from build123d import *

# Parameters (mm, degrees)
CHAMFER1_SIZE                   = 2
BOSS_EXTRUDE1_DEPTH             = 70
CHAMFER2_SIZE                   = 14
SKETCH3_R                       = 5
CUT_EXTRUDE1_DEPTH              = 70
CIRPATTERN1_COUNT               = 4
CHAMFER2_OF_CIRPATTERN1_SIZE    = 14
CUT_EXTRUDE2_START              = 70
CUT_EXTRUDE2_DEPTH              = 70
CUT_EXTRUDE3_DEPTH              = 70
CIRPATTERN2_COUNT               = 2
CIRPATTERN2_ANGLE               = 10
CIRPATTERN2_THE_OTHER_WAY_COUNT = 2
CIRPATTERN2_THE_OTHER_WAY_ANGLE = 10
CIRPATTERN3_COUNT               = 4
CIRPATTERN3_COPY_1_DEPTH        = 70
CIRPATTERN3_COPY_2_DEPTH        = 70
CIRPATTERN3_COPY_3_DEPTH        = 70
CIRPATTERN3_COPY_4_DEPTH        = 70
CIRPATTERN3_COPY_5_DEPTH        = 70
CIRPATTERN3_COPY_6_DEPTH        = 70
CUT_SWEEP2_PROFILE_R            = 0.5
CUT_SWEEP3_PROFILE_R            = 0.5
CUT_EXTRUDE4_START              = -10
SKETCH27_R                      = 37.5
CUT_EXTRUDE4_DEPTH              = 10


with BuildPart() as part:
    # Sketch1 → Revolve1 (revolve)
    with BuildSketch(Plane.XY, mode=Mode.PRIVATE) as revolve1_sk:
        Polygon((0, 0), (-50, 0), (-50, 28), (-37.5, 28), (-37.5, 31), (-5, 31), (-5, 41), (0, 41), align=None)
    revolve(revolve1_sk.sketch.rotate(Axis((0, 0, 0), (0, 1, 0)), 270), axis=Axis((0, 0, 0), (0, 1, 0)))

    # Chamfer1
    chamfer1_edges = [part.edges().sort_by_distance(p)[0] for p in [
        (0, 31, 37.5),
        (0, 28, 50),
    ]]
    chamfer(chamfer1_edges, length=CHAMFER1_SIZE)

    # Sketch2 → Boss-Extrude1 (add)
    with BuildSketch(Plane.XY):
        Polygon((12.5, 0), (-12.5, 0), (-12.5, 26), (-10.5, 26), (-10.5, 2), (10.5, 2), (10.5, 26), (12.5, 26), align=None)
    boss_extrude1 = extrude(amount=BOSS_EXTRUDE1_DEPTH)

    # Chamfer2
    chamfer2_edges = [part.edges().sort_by_distance(p)[0] for p in [
        (-11.5, 26, 70),
        (11.5, 26, 70),
    ]]
    chamfer(chamfer2_edges, length=CHAMFER2_SIZE)

    # Sketch3 → Cut-Extrude1 (cut)
    with BuildSketch(Plane(origin=(0, 31, 0), x_dir=(1, 0, 0), z_dir=(0, 1, 0))):
        with Locations(Location((0, -60, 0), (0, 0, 270))):
            Circle(SKETCH3_R)
    cut_extrude1 = extrude(amount=-CUT_EXTRUDE1_DEPTH, mode=Mode.SUBTRACT)

    # CirPattern1: Boss-Extrude1, Cut-Extrude1 ×4 about axis
    cirpattern1_axis = Axis((0, 0, 0), (0, 1, 0))
    add([boss_extrude1.rotate(cirpattern1_axis, i * 360 / CIRPATTERN1_COUNT) for i in range(1, CIRPATTERN1_COUNT)])
    add([cut_extrude1.rotate(cirpattern1_axis, i * 360 / CIRPATTERN1_COUNT) for i in range(1, CIRPATTERN1_COUNT)], mode=Mode.SUBTRACT)

    # Chamfer2 of CirPattern1
    chamfer2_of_cirpattern1_edges = [part.edges().sort_by_distance(p)[0] for p in [
        (70, 26, 11.5),
        (70, 26, -11.5),
        (11.5, 26, -70),
        (-11.5, 26, -70),
        (-70, 26, -11.5),
        (-70, 26, 11.5),
    ]]
    chamfer(chamfer2_of_cirpattern1_edges, length=CHAMFER2_OF_CIRPATTERN1_SIZE)

    # Sketch4 → Cut-Extrude2 (cut)
    with BuildSketch(Plane(origin=(0, 0, 0), x_dir=(1, 0, 0), z_dir=(0, 1, 0)).offset(CUT_EXTRUDE2_START)):
        with BuildLine():
            Line((23.02513458, -42.117017672), (23.12024219, -44.333445626))
            ThreePointArc((23.12024219, -44.333445626), (35.355339059, -35.355339059), (44.333445626, -23.12024219))
            Line((44.333445626, -23.12024219), (42.117017672, -23.02513458))
            ThreePointArc((42.117017672, -23.02513458), (33.941125497, -33.941125497), (23.02513458, -42.117017672))
        make_face()
    cut_extrude2 = extrude(amount=-CUT_EXTRUDE2_DEPTH, mode=Mode.SUBTRACT)

    # Sketch5 → Cut-Extrude3 (cut)
    with BuildSketch(Plane(origin=(0, 0, 0), x_dir=(1, 0, 0), z_dir=(0, 1, 0))):
        Polygon((30.939685977, -33.941125497), (34.034072747, -36.941125497), (36.942565017, -33.941125497), (33.848178247, -30.941125497), align=None)
    cut_extrude3 = extrude(amount=CUT_EXTRUDE3_DEPTH, mode=Mode.SUBTRACT)

    # CirPattern2: Cut-Extrude3 ×2 about axis
    cirpattern2_axis = Axis((0, 0, 0), (0, 1, 0))
    for i in range(1, CIRPATTERN2_COUNT):
        add(cut_extrude3.rotate(cirpattern2_axis, i * CIRPATTERN2_ANGLE / (CIRPATTERN2_COUNT - 1)), mode=Mode.SUBTRACT)

    # CirPattern2 the other way: Cut-Extrude3 ×2 about axis
    cirpattern2_the_other_way_axis = Axis((0, 0, 0), (0, -1, 0))
    for i in range(1, CIRPATTERN2_THE_OTHER_WAY_COUNT):
        add(cut_extrude3.rotate(cirpattern2_the_other_way_axis, i * CIRPATTERN2_THE_OTHER_WAY_ANGLE / (CIRPATTERN2_THE_OTHER_WAY_COUNT - 1)), mode=Mode.SUBTRACT)

    # CirPattern3: Cut-Extrude2, Cut-Extrude3 ×4 about axis
    cirpattern3_axis = Axis((0, 0, 0), (0, 1, 0))
    add([cut_extrude2.rotate(cirpattern3_axis, i * 360 / CIRPATTERN3_COUNT) for i in range(1, CIRPATTERN3_COUNT)], mode=Mode.SUBTRACT)
    add([cut_extrude3.rotate(cirpattern3_axis, i * 360 / CIRPATTERN3_COUNT) for i in range(1, CIRPATTERN3_COUNT)], mode=Mode.SUBTRACT)

    # CirPattern3 copy 1 sketch → CirPattern3 copy 1 (cut)
    with BuildSketch(Plane(origin=(0, 0, 0), x_dir=(-0.1736481776669307, 0, -0.984807753012208), z_dir=(0, 1, 0))):
        Polygon((30.939685977, -33.941125497), (34.034072747, -36.941125497), (36.942565017, -33.941125497), (33.848178247, -30.941125497), align=None)
    extrude(amount=CIRPATTERN3_COPY_1_DEPTH, mode=Mode.SUBTRACT)

    # CirPattern3 copy 2 sketch → CirPattern3 copy 2 (cut)
    with BuildSketch(Plane(origin=(0, 0, 0), x_dir=(-0.984807753012208, 0, 0.17364817766693064), z_dir=(0, 1, 0))):
        Polygon((30.939685977, -33.941125497), (34.034072747, -36.941125497), (36.942565017, -33.941125497), (33.848178247, -30.941125497), align=None)
    extrude(amount=CIRPATTERN3_COPY_2_DEPTH, mode=Mode.SUBTRACT)

    # CirPattern3 copy 3 sketch → CirPattern3 copy 3 (cut)
    with BuildSketch(Plane(origin=(0, 0, 0), x_dir=(0.17364817766693055, 0, 0.984807753012208), z_dir=(0, 1, 0))):
        Polygon((30.939685977, -33.941125497), (34.034072747, -36.941125497), (36.942565017, -33.941125497), (33.848178247, -30.941125497), align=None)
    extrude(amount=CIRPATTERN3_COPY_3_DEPTH, mode=Mode.SUBTRACT)

    # CirPattern3 copy 4 sketch → CirPattern3 copy 4 (cut)
    with BuildSketch(Plane(origin=(0, 0, 0), x_dir=(0.1736481776669308, 0, -0.984807753012208), z_dir=(0, 1, 0))):
        Polygon((30.939685977, -33.941125497), (34.034072747, -36.941125497), (36.942565017, -33.941125497), (33.848178247, -30.941125497), align=None)
    extrude(amount=CIRPATTERN3_COPY_4_DEPTH, mode=Mode.SUBTRACT)

    # CirPattern3 copy 5 sketch → CirPattern3 copy 5 (cut)
    with BuildSketch(Plane(origin=(0, 0, 0), x_dir=(-0.984807753012208, 0, -0.17364817766693086), z_dir=(0, 1, 0))):
        Polygon((30.939685977, -33.941125497), (34.034072747, -36.941125497), (36.942565017, -33.941125497), (33.848178247, -30.941125497), align=None)
    extrude(amount=CIRPATTERN3_COPY_5_DEPTH, mode=Mode.SUBTRACT)

    # CirPattern3 copy 6 sketch → CirPattern3 copy 6 (cut)
    with BuildSketch(Plane(origin=(0, 0, 0), x_dir=(-0.17364817766693094, 0, 0.984807753012208), z_dir=(0, 1, 0))):
        Polygon((30.939685977, -33.941125497), (34.034072747, -36.941125497), (36.942565017, -33.941125497), (33.848178247, -30.941125497), align=None)
    extrude(amount=CIRPATTERN3_COPY_6_DEPTH, mode=Mode.SUBTRACT)

    # Cut-Sweep2: sweep along a path in Sketch15
    with BuildLine(Plane(origin=(0, 28, 0), x_dir=(1, 0, 0), z_dir=(0, 1, 0))) as cut_sweep2_path:
        CenterArc((0, 0), 44, 0, 360)
    # Cut-Sweep2 profile (on start of the path) → Cut-Sweep2 (sweep, cut)
    with BuildSketch(Plane(origin=(44, 28, 0), x_dir=(-1, 0, 0), z_dir=(0, 0, -1))):
        Circle(CUT_SWEEP2_PROFILE_R)
    sweep(path=cut_sweep2_path.line, mode=Mode.SUBTRACT)

    # Cut-Sweep3: sweep along a path in Sketch14
    with BuildLine(Plane(origin=(0, 28, 0), x_dir=(1, 0, 0), z_dir=(0, 1, 0))) as cut_sweep3_path:
        CenterArc((0, 0), 41, 0, 360)
    # Cut-Sweep3 profile (on start of the path) → Cut-Sweep3 (sweep, cut)
    with BuildSketch(Plane(origin=(41, 28, 0), x_dir=(-1, 0, 0), z_dir=(0, 0, -1))):
        Circle(CUT_SWEEP3_PROFILE_R)
    sweep(path=cut_sweep3_path.line, mode=Mode.SUBTRACT)

    # Sketch27 → Cut-Extrude4 (cut)
    with BuildSketch(Plane.XZ.offset(CUT_EXTRUDE4_START)):
        with Locations(Location((0, 0, 0), (0, 0, 270))):
            Circle(SKETCH27_R)
    extrude(amount=CUT_EXTRUDE4_DEPTH, mode=Mode.SUBTRACT)


solid = part.part
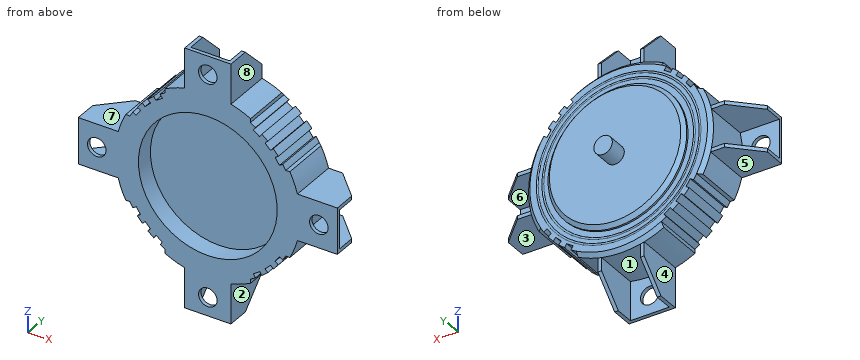
The listing builds one solid part. Answer for the finished solid, in the listing's coordinates (mm). Face numbers are marked on the shaded views. A direction names the side the tool comes from. Round coordinates to 2 decimals unless told otherwise and drop trailing zeros. Order: outer loops, then holes, each group sorted by start corner. A loop starts at its lowest first (then second) coordinate and runs counter-clockwise, first axis right, second up. Notation, with made-up numbers: (-8, 41) - (10, 41) arc R19 cw to (10, 61) - close; hole circle Ø11 at (55, 73.25). An arc over 180 degrees is marked (long way). Write item = value, one per line. Start each with the question number.
1) Section B-B, the plane x = 0 is taken. Count the separate pieces of the cut face and the enclosed holes in it, plus the area to 3 significant figures.
2) Section D-D, the plane y = 37 is taken. Write down the section's boundary in (x, z).
3) Section A-A, the plane x = -60 is taken. Write down the section's boundary in (y, z), plus the area to 3 significant figures.
4) Straight lines are drawn through the part: L1, parallel to Z at x = -57, y = 12; L2, parallel to Z at x = -60, y = 1.1. For each, find the intervals that lie inside material, in ascending order.
5) For a pull along X with two mould halves and no side action, classify the marked faces 1, 2, 3 and 4 as released by +X, released by -X, zero draft, split by the parting line, or undercut.
6) For the marked faces 5, 6, 7 and 8, determine the directions among +Z, -Z, +X, -X, +Y, -Y from which every point of the face is accessible in a straight line to the end or side of a thin tool.
7) Given pin 1 (1.5 mm diameter, centred on y = 33.5, z = 26, fed in from -X); pin 2 (11 mm diameter, centred on y = 18.5, z = 62.5, fed in from +X); pin 3 (12 mm diameter, centred on x = 9.5, y = 36, fed in from -Z); pin 4 (1.5 mm diameter, centred on x = -15, z = 21.5, fed in from -Y), each flat-ended and moving along its own axis, determine where each tip first touches the part or whether it passes through.
Results list:
q1.separate_pieces = 3
q1.enclosed_holes = 0
q1.area = 2,410 mm^2
q2.outline = circle Ø10 at (0, 0)
q3.outline = (0, -12.5) - (22, -12.5) - (22, -10.5) - (2, -10.5) - (2, -5) - (0, -5) - close; (0, 5) - (2, 5) - (2, 10.5) - (22, 10.5) - (22, 12.5) - (0, 12.5) - close
q3.area = 110 mm^2
q4.L1 = -12.5 to -10.5, 10.5 to 12.5
q4.L2 = -12.5 to -5, 5 to 12.5
q5.face_1 = undercut
q5.face_2 = released by +X
q5.face_3 = zero draft
q5.face_4 = released by -X
q6.face_5 = -Z, -X, +Y, -Y
q6.face_6 = +X, +Y
q6.face_7 = +Z, -X, +Y, -Y
q6.face_8 = +Z, +X, +Y, -Y
q7.pin_1 = through
q7.pin_2 = 12.5
q7.pin_3 = -35.42
q7.pin_4 = 10
